The listing builds one solid part. Answer for the finished solid, in the listing's coordinates (mm). A direction names the side the tool comes from. Coordinates: 2 decimals unless noted, no trailing zeros. Order: outer loops, then holes, each group sorted by start corner. A loop starts at its lowest first (then second) coordinate and runs counter-clockwise, first axis right, second up. Notation, with made-up numbers: (72, -37.75) - (84, -37.75) arc R11 cw to (84, -23.75) - close; hole circle Ø5 at (52, 71.25). An arc over 180 degrees is marked (long way). Use one line per item in the form item = value. Start each with the question number.
Item 1: Section D-D, the plane y = -9 is taken. Write down the section's boundary in (x, z) (3 decimals).
Item 2: Section C-C, the plane y = 8 is taken. Write down the section's boundary in (x, z) (3 decimals), and give its area (3 significant figures).
Item 3: Consider line 1 along Z through (x, y) = (20, 16) (3 decimals); line 2 along Z through (x, y) = (4, -5) (3 decimals); line 3 along Y through (x, z) = (-19.5, -19). Determine where each line is inside the solid, lowest interval first. Write a range as [from, to].
Item 4: The mould has two halves that part along Z. Classify faces 5 (the cylindrical face through (18.928, 34.186, 3.333)), 6 (the flat face through (20, 20, -27)): released by +Z, released by -Z, zero draft, split by the parting line, or undercut.
Item 5: A tool of negligible diameter and unlimited length cuts with its end or side. For faces 1 (the flat face through (-20, 12, -16.875)), 2 (the flat face through (20, 2, -24.875)), 3 (the flat face through (-17.146, 38.696, -0.848)), 4 (the flat face through (-13.9, -2, -14)), from which of +Z, -Z, +X, -X, +Y, -Y can it reach the whole face along a straight path? Write none if from no direction.
Item 6: Section A-A, the plane y = 32.6 is taken. Count the separate pieces of the cut face and the enclosed holes in it, and give its area (3 significant figures).
Item 7: Each of these flat-tipped pins is pushed along its axis until it touches: pin 1 Ø3.5 at (x, z) = (-5, -39.875) entering from +Y; pin 2 Ø2 at (x, y) = (12.5, 29.5) entering from -Z (3 decimals); pin 3 Ø5 at (x, z) = (13.5, -24.5) entering from -Y. Where does it stop, or does it pass through?
from build123d import *

# Parameters (mm, degrees)
EXTRUDE_1_DEPTH      = 40
SKETCH_1_3_W         = 33.8
SKETCH_1_3_H         = 23.75
SKETCH_1_3_R         = 1.6
EXTRUDE_2_DEPTH      = 8
SKETCH_4_R           = 1.6
CUT_EXTRUDE_1_DEPTH  = 82.129560735
SKETCH_8_W           = 4
SKETCH_8_H           = 43
EXTRUDE_3_DEPTH      = 20
EXTRUDE_START        = 3
SKETCH_11_R          = 1.6
EXTRUDE_5_DEPTH      = 3
SKETCH_12_R          = 1.6
EXTRUDE_6_DEPTH      = 3
FILLET_4_R           = 20
SKETCH_10_R          = 1.6
CUT_EXTRUDE_4_DEPTH  = 85.377755511
CHAMFER_1_SIZE       = 0.5
CHAMFER_1_SIZE2      = 2.572277008
HOLE_WIZARD_M3_1_D   = 3.2
SKETCH_14_W          = 5
SKETCH_14_H          = 48.410238409
CUT_EXTRUDE_6_DEPTH  = 10
CUT_EXTRUDE_11_REACH = 80.166
SKETCH_22_W          = 5.804167704
SKETCH_22_H          = 22.848634954
CHAMFER_2_SIZE       = 0.5
SKETCH_13_W          = 13
SKETCH_13_H          = 5
CUT_EXTRUDE_5_DEPTH  = 53
SKETCH_17_R          = 3
CUT_EXTRUDE_8_DEPTH  = 85.377755511
SKETCH_19_W          = 25
SKETCH_19_H          = 25
EXTRUDE_7_DEPTH      = 7
SKETCH_20_W          = 15.2
SKETCH_20_H          = 15.2
EXTRUDE_8_DEPTH      = 2
CHAMFER_3_SIZE       = 2
SKETCH_21_R          = 1.6
CUT_EXTRUDE_10_DEPTH = 74.52534002
SKETCH_18_R          = 3
CUT_EXTRUDE_9_DEPTH  = 6
CHAMFER_5_SIZE       = 7


with BuildPart() as part:
    # 草图1 → 凸台-拉伸1 (new body)
    with BuildSketch(Plane(origin=(0, 0, 0), x_dir=(1, 0, 0), z_dir=(0, 1, 0))):
        Polygon((-16.9, -9.875), (-16.9, 13.875), (-20.9, 13.875), (-20.9, -13.875), (20.9, -13.875), (20.9, 13.875), (16.9, 13.875), (16.9, -9.875), align=None)
    extrude(amount=EXTRUDE_1_DEPTH)

    # 草图1<3> → 凸台-拉伸2 (add)
    # profile 1 of 3: a face of its own
    with BuildSketch(Plane(origin=(0, 0, 0), x_dir=(1, 0, 0), z_dir=(0, 1, 0))):
        with Locations((0, 2)):
            Rectangle(SKETCH_1_3_W, SKETCH_1_3_H)
    # profile 2 of 3: a face of its own
    with BuildSketch(Plane(origin=(0, 0, 0), x_dir=(1, 0, 0), z_dir=(0, 1, 0))):
        Polygon((-20.9, 13.875), (-16.9, 13.875), (16.9, 13.875), (20.9, 13.875), (20.9, 56.875), (-20.9, 56.875), align=None)
        with Locations(Location((-5, 29.875, 0), (0, 0, 270))):
            Circle(SKETCH_1_3_R, mode=Mode.SUBTRACT)
        with Locations(Location((-5, 39.875, 0), (0, 0, 270))):
            Circle(SKETCH_1_3_R, mode=Mode.SUBTRACT)
        with Locations(Location((5, 29.875, 0), (0, 0, 270))):
            Circle(SKETCH_1_3_R, mode=Mode.SUBTRACT)
        with Locations(Location((5, 39.875, 0), (0, 0, 270))):
            Circle(SKETCH_1_3_R, mode=Mode.SUBTRACT)
    # profile 3 of 3: a face of its own
    with BuildSketch(Plane(origin=(0, 0, 0), x_dir=(1, 0, 0), z_dir=(0, 1, 0))):
        Polygon((-16.9, -9.875), (-16.9, 13.875), (-20.9, 13.875), (-20.9, -13.875), (20.9, -13.875), (20.9, 13.875), (16.9, 13.875), (16.9, -9.875), align=None)
    extrude(amount=-EXTRUDE_2_DEPTH)

    # 草图4 → 切除-拉伸1 (cut, through all)
    with BuildSketch(Plane(origin=(20.9, 0, 0), x_dir=(0, 0, -1), z_dir=(1, 0, 0))):
        with Locations((-3.125, 16.6)):
            Circle(SKETCH_4_R)
        with Locations((-3.125, 32.6)):
            Circle(SKETCH_4_R)
    extrude(amount=-CUT_EXTRUDE_1_DEPTH, mode=Mode.SUBTRACT)

    # 草图8 → 凸台-拉伸3 (add)
    with BuildSketch(Plane(origin=(0, 0, 0), x_dir=(1, 0, 0), z_dir=(0, 1, 0))):
        with Locations((18.9, 35.375)):
            Rectangle(SKETCH_8_W, SKETCH_8_H)
        with Locations((-18.9, 35.375)):
            Rectangle(SKETCH_8_W, SKETCH_8_H)
    extrude(amount=EXTRUDE_3_DEPTH)

    # 草图11 → 凸台-拉伸5 (add)
    with BuildSketch(Plane(origin=(20.9, 0, 0), x_dir=(0, 0, -1), z_dir=(1, 0, 0)).offset(EXTRUDE_START)):
        Polygon((-13.875, 40), (13.875, 40), (13.875, 20), (56.875, 20), (56.875, -8), (-13.875, -8), align=None)
        with Locations((-3.125, 32.6)):
            Circle(SKETCH_11_R, mode=Mode.SUBTRACT)
        with Locations((-3.125, 16.6)):
            Circle(SKETCH_11_R, mode=Mode.SUBTRACT)
    extrude(amount=-EXTRUDE_5_DEPTH)

    # 草图12 → 凸台-拉伸6 (add)
    with BuildSketch(Plane.ZY.offset(20.9)):
        Polygon((-13.875, 40), (13.875, 40), (13.875, -8), (-56.875, -8), (-56.875, 20), (-13.875, 20), align=None)
        with Locations(Location((3.125, 32.6, 0), (0, 0, 180))):
            Circle(SKETCH_12_R, mode=Mode.SUBTRACT)
        with Locations(Location((3.125, 16.6, 0), (0, 0, 180))):
            Circle(SKETCH_12_R, mode=Mode.SUBTRACT)
    extrude(amount=EXTRUDE_6_DEPTH)

    # 圆角4
    fillet_4_edges = [part.edges().sort_by_distance(p)[0] for p in [
        (20.4, 20, -56.875),
        (-20.4, 20, -56.875),
    ]]
    fillet(fillet_4_edges, radius=FILLET_4_R)

    # 草图10 → 切除-拉伸4 (cut, through all)
    with BuildSketch(Plane.ZY.offset(23.9)):
        with Locations((-28.875, 16.6)):
            Circle(SKETCH_10_R)
    extrude(amount=-CUT_EXTRUDE_4_DEPTH, mode=Mode.SUBTRACT)

    # 倒角1
    chamfer_1_edges = [part.edges().sort_by_distance(p)[0] for p in [
        (-16.9, 40, -2),
        (16.9, 40, -2),
    ]]
    chamfer_1_side = [part.faces().sort_by_distance(p)[0] for p in [
        (-17.452711724, 40, -2),
    ]]
    chamfer(chamfer_1_edges, length=CHAMFER_1_SIZE, length2=CHAMFER_1_SIZE2, reference=chamfer_1_side[0])

    # M3 间隙孔1 (through all)
    with Locations(Plane.XY.offset(13.875)):
        with Locations((-10, 32.6), (-10, 16.6), (10, 16.6), (10, 32.6)):
            Hole(HOLE_WIZARD_M3_1_D / 2)

    # 草图14 → 切除-拉伸6 (cut)
    with BuildSketch(Plane(origin=(23.9, 0, 0), x_dir=(0, 0, -1), z_dir=(1, 0, 0))):
        with Locations((14.375, 20.3953107)):
            Rectangle(SKETCH_14_W, SKETCH_14_H)
    cut_extrude_6 = extrude(amount=-CUT_EXTRUDE_6_DEPTH, mode=Mode.SUBTRACT)

    # 切除-拉伸11: up to this face of the body (flat: up to its plane)
    cut_extrude_11_end = Plane(part.part.faces().sort_by_distance((18.9, -3.809808505, -14.375))[0])
    # 草图22 → 切除-拉伸11 (cut, up to the picked face)
    with BuildSketch(Plane(origin=(0, 40, 0), x_dir=(1, 0, 0), z_dir=(0, 1, 0)), mode=Mode.PRIVATE) as cut_extrude_11_sk1:
        with Locations((23.802083852, 3.549317477)):
            Rectangle(SKETCH_22_W, SKETCH_22_H)
    cut_extrude_11_tool1 = split(extrude(cut_extrude_11_sk1.sketch, amount=-CUT_EXTRUDE_11_REACH, mode=Mode.PRIVATE), bisect_by=cut_extrude_11_end, keep=Keep.BOTH, mode=Mode.PRIVATE)
    cut_extrude_11 = cut_extrude_11_tool1.solids().sort_by(Axis((23.802084, 40, -3.549317), (0, -1, 0)))[0]
    add(cut_extrude_11, mode=Mode.SUBTRACT)

    # 镜向1: 切除-拉伸6, 切除-拉伸11 across plane
    add(cut_extrude_6.mirror(Plane(origin=(0, 0, 0), x_dir=(0, 0, 1), z_dir=(1, 0, 0))), mode=Mode.SUBTRACT)
    add(cut_extrude_11.mirror(Plane(origin=(0, 0, 0), x_dir=(0, 0, 1), z_dir=(1, 0, 0))), mode=Mode.SUBTRACT)

    # 倒角2
    chamfer_2_edges = [part.edges().sort_by_distance(p)[0] for p in [
        (-23.9, 16, 13.875),
        (0, -8, 13.875),
        (0, 40, 13.875),
        (23.9, 16, 13.875),
    ]]
    chamfer(chamfer_2_edges, length=CHAMFER_2_SIZE)

    # 草图13 → 切除-拉伸5 (cut)
    with BuildSketch(Plane(origin=(23.9, 0, 0), x_dir=(0, 0, -1), z_dir=(1, 0, 0))):
        with Locations((18.375, 2.5)):
            Rectangle(SKETCH_13_W, SKETCH_13_H)
    extrude(amount=-CUT_EXTRUDE_5_DEPTH, mode=Mode.SUBTRACT)

    # 草图17 → 切除-拉伸8 (cut, through all)
    with BuildSketch(Plane(origin=(23.9, 0, 0), x_dir=(0, 0, -1), z_dir=(1, 0, 0))):
        with Locations((5.875, 18.5)):
            Circle(SKETCH_17_R)
    extrude(amount=-CUT_EXTRUDE_8_DEPTH, mode=Mode.SUBTRACT)

    # 草图19 → 凸台-拉伸7 (add)
    with BuildSketch(Plane.XZ.offset(8)):
        with Locations((0, -34.875)):
            Rectangle(SKETCH_19_W, SKETCH_19_H)
    extrude(amount=EXTRUDE_7_DEPTH)

    # 草图20 → 凸台-拉伸8 (add)
    with BuildSketch(Plane.XZ.offset(15)):
        with Locations((0, -34.875)):
            Rectangle(SKETCH_20_W, SKETCH_20_H)
    extrude(amount=EXTRUDE_8_DEPTH)

    # 倒角3
    chamfer_3_edges = [part.edges().sort_by_distance(p)[0] for p in [
        (7.6, -15, -34.875),
        (0, -15, -42.475),
        (-7.6, -15, -34.875),
        (0, -15, -27.275),
    ]]
    chamfer(chamfer_3_edges, length=CHAMFER_3_SIZE - 0.0001)  # a hair under: the kernel refuses the full size

    # 草图21 → 切除-拉伸10 (cut, through all)
    with BuildSketch(Plane(origin=(0, 0, 0), x_dir=(1, 0, 0), z_dir=(0, 1, 0))):
        with Locations(Location((-5, 39.875, 0), (0, 0, 270))):
            Circle(SKETCH_21_R)
        with Locations(Location((5, 39.875, 0), (0, 0, 270))):
            Circle(SKETCH_21_R)
        with Locations(Location((5, 29.875, 0), (0, 0, 270))):
            Circle(SKETCH_21_R)
        with Locations(Location((-5, 29.875, 0), (0, 0, 270))):
            Circle(SKETCH_21_R)
    extrude(amount=-CUT_EXTRUDE_10_DEPTH, mode=Mode.SUBTRACT)

    # 草图18 → 切除-拉伸9 (cut)
    with BuildSketch(Plane(origin=(0, 0, 0), x_dir=(1, 0, 0), z_dir=(0, 1, 0))):
        with Locations(Location((-5, 39.875, 0), (0, 0, 270))):
            Circle(SKETCH_18_R)
        with Locations(Location((5, 39.875, 0), (0, 0, 270))):
            Circle(SKETCH_18_R)
        with Locations(Location((5, 29.875, 0), (0, 0, 270))):
            Circle(SKETCH_18_R)
        with Locations(Location((-5, 29.875, 0), (0, 0, 270))):
            Circle(SKETCH_18_R)
    extrude(amount=-CUT_EXTRUDE_9_DEPTH, mode=Mode.SUBTRACT)

    # 倒角5
    chamfer_5_edges = [part.edges().sort_by_distance(p)[0] for p in [
        (-12.5, -8, -34.875),
        (0, -8, -47.375),
        (12.5, -8, -34.875),
        (0, -8, -22.375),
    ]]
    chamfer(chamfer_5_edges, length=CHAMFER_5_SIZE - 0.0001)  # a hair under: the kernel refuses the full size


solid = part.part
Response:
q1.outline = (-18.5, -53.375) - (18.5, -53.375) - (18.5, -16.375) - (-18.5, -16.375) - close; hole circle Ø3.2 at (-5, -39.875); hole circle Ø3.2 at (-5, -29.875); hole circle Ø3.2 at (5, -39.875); hole circle Ø3.2 at (5, -29.875)
q2.outline = (-23.9, -55.205) - (-16.9, -55.205) - (-16.9, -16.875) - (-23.9, -16.875) - close; (-23.9, 7.875) - (-20.9, 7.875) - (-20.9, -11.875) - (-16.9, -11.875) - (-16.9, 9.875) - (16.9, 9.875) - (16.9, -11.875) - (20.9, -11.875) - (20.9, 7.875) - (23.9, 7.875) - (23.9, 13.375) - (23.4, 13.875) - (-23.4, 13.875) - (-23.9, 13.375) - close; (16.9, -55.205) - (23.9, -55.205) - (23.9, -16.875) - (16.9, -16.875) - close
q2.area = 914 mm2
q3.line_1 = [-48.875, -30.358], [-27.392, -16.875], [-11.875, -7.533], [-4.217, 1.642], [4.608, 13.875]
q3.line_2 = [-56.875, -42.703], [-37.047, -32.703], [-27.047, 13.875]
q3.line_3 = [-8, 0], [5, 20]
q4.face_5 = undercut
q4.face_6 = zero draft
q5.face_1 = +X, -X, +Y
q5.face_2 = +X, -X
q5.face_3 = -Z, +Y
q5.face_4 = -X, +Y
q6.separate_pieces = 5
q6.enclosed_holes = 0
q6.area = 326 mm2
q7.pin_1 = -6
q7.pin_2 = 9.875
q7.pin_3 = -15
